```python
from build123d import *

# Parameters (mm, degrees)
F0_R     = 6.35
F1_DEPTH = 25.4
F2_SIZE  = 6.35
F3_W     = 63.5
F3_H     = 19.05
F4_DEPTH = 95.25
F5_R     = 6.35
F7_DEPTH = 50.801


with BuildPart() as f1:
    # F0 (on Top) → F1 (new body)
    with BuildSketch(Plane.XY):
        with BuildLine():
            ThreePointArc((0, 15.875), (4.6496798487, 4.6496798487), (15.875, 0))
            Line((15.875, 0), (60.325, 0))
            ThreePointArc((60.325, 0), (71.5503201513, 4.6496798487), (76.2, 15.875))
            Line((76.2, 15.875), (76.2, 85.725))
            ThreePointArc((76.2, 85.725), (71.5503201513, 96.9503201513), (60.325, 101.6))
            Line((60.325, 101.6), (15.875, 101.6))
            ThreePointArc((15.875, 101.6), (4.6496798487, 96.9503201513), (0, 85.725))
            Line((0, 85.725), (0, 15.875))
        make_face()
        with Locations((15.875, 15.875)):
            Circle(F0_R, mode=Mode.SUBTRACT)
        with Locations((60.325, 15.875)):
            Circle(F0_R, mode=Mode.SUBTRACT)
        with Locations((15.875, 85.725)):
            Circle(F0_R, mode=Mode.SUBTRACT)
        with Locations((60.325, 85.725)):
            Circle(F0_R, mode=Mode.SUBTRACT)
    extrude(amount=F1_DEPTH)

    # F2
    f2_edges = [f1.edges().sort_by_distance(p)[0] for p in [
        (38.1, 0, 25.4),
        (0, 50.8, 25.4),
        (4.64968, 4.64968, 25.4),
        (71.55032, 4.64968, 25.4),
        (76.2, 50.8, 25.4),
        (71.55032, 96.95032, 25.4),
        (38.1, 101.6, 25.4),
        (4.64968, 96.95032, 25.4),
    ]]
    chamfer(f2_edges, length=F2_SIZE)

    # F3 (on face) → F4 (join)
    with BuildSketch(Plane.XY.offset(25.4)):
        with Locations((38.1, 60.325)):
            Rectangle(F3_W, F3_H)
    extrude(amount=F4_DEPTH)

    # F5
    f5_edges = [f1.edges().sort_by_distance(p)[0] for p in [
        (38.1, 50.8, 25.4),
        (38.1, 69.85, 25.4),
    ]]
    fillet(f5_edges, radius=F5_R)

    # F6 (on face) → F7 (cut, through all)
    with BuildSketch(Plane.XZ.offset(-50.8)):
        with BuildLine():
            Line((6.35, 120.65), (6.35, 61.0775296334))
            ThreePointArc((6.35, 61.0775296334), (9.7019366858, 75.2765612905), (19.05, 86.4775296334))
            Line((19.05, 86.4775296334), (19.05, 120.65))
            Line((19.05, 120.65), (6.35, 120.65))
        make_face()
        with BuildLine():
            ThreePointArc((57.15, 61.0775296334), (38.1, 80.1275296334), (19.05, 61.0775296334))
            Line((19.05, 61.0775296334), (38.1, 61.0775296334))
            Line((38.1, 61.0775296334), (38.1, 42.0275296334))
            ThreePointArc((38.1, 42.0275296334), (51.5703841816, 47.6071454518), (57.15, 61.0775296334))
        make_face()
        with BuildLine():
            Line((19.05, 86.4775296334), (19.05, 61.0775296334))
            ThreePointArc((19.05, 61.0775296334), (38.1, 80.1275296334), (57.15, 61.0775296334))
            Line((57.15, 61.0775296334), (57.15, 86.4775296334))
            ThreePointArc((57.15, 86.4775296334), (38.1, 92.8275296334), (19.05, 86.4775296334))
        make_face()
        with BuildLine():
            Line((38.1, 61.0775296334), (19.05, 61.0775296334))
            ThreePointArc((19.05, 61.0775296334), (24.6296158184, 47.6071454518), (38.1, 42.0275296334))
            Line((38.1, 42.0275296334), (38.1, 61.0775296334))
        make_face()
        with BuildLine():
            Line((19.05, 120.65), (19.05, 86.4775296334))
            ThreePointArc((19.05, 86.4775296334), (38.1, 92.8275296334), (57.15, 86.4775296334))
            Line((57.15, 86.4775296334), (57.15, 120.65))
            Line((57.15, 120.65), (19.05, 120.65))
        make_face()
        with BuildLine():
            ThreePointArc((57.15, 86.4775296334), (66.4980633142, 75.2765612905), (69.85, 61.0775296334))
            Line((69.85, 61.0775296334), (69.85, 120.65))
            Line((69.85, 120.65), (57.15, 120.65))
            Line((57.15, 120.65), (57.15, 86.4775296334))
        make_face()
    extrude(amount=-F7_DEPTH, mode=Mode.SUBTRACT)


solid = f1.part
```
Source: CAD feature listing. Evaluate the final solid. Frame: model axes, mm. A direction names the side the tool comes from. Coordinates: 2 decimals unless noted, no trailing zeros. Order: outer loops, then holes, each group sorted by start corner. A loop starts at its lowest first (then second) coordinate and runs counter-clockwise, first axis right, second up. Notation, with made-up numbers: (-16, -8) - (7, -8) arc R22 cw to (7, 5) - close; hole circle Ø1 at (-22, 28.5). An arc over 180 degrees is marked (long way). One line per item, written item: value.
1) Cut plane D-D on x = 23.5. Output: boundary loops of the cut face in (y, z).
Computed values:
outline: (0, 0) - (101.6, 0) - (101.6, 19.05) - (95.25, 25.4) - (76.2, 25.4) arc R6.35 cw to (69.85, 31.75) - (69.85, 48.84) - (50.8, 48.84) - (50.8, 31.75) arc R6.35 cw to (44.45, 25.4) - (6.35, 25.4) - (0, 19.05) - close
2) Mould query, pull axis X, two halves, no side actions, for faces 1 (the face through (76.2, 50, 9)), 2 (the face through (38.41, 98.38, 22.27)), 3 (the face through (9.61, 60.19, 75.09)), 4 (the face through (66.19, 13.44, 12.52)). Classes: released by +X, released by -X, zero draft, split by the parting line, or undercut.
Computed values:
face 1: released by +X
face 2: zero draft
face 3: released by -X
face 4: undercut
3) Ray query, line 1 (X direction, y = 21, z = 22); line 2 (Z direction, x = 73, y = 55.5); line 3 (X direction, y = 62.5, z = 48). Return the intervals inside material, ascending. Write a range as [from, to].
Computed values:
line 1: x = [2.95, 12.13], [19.62, 56.58], [64.07, 73.25]
line 2: z = [0, 22.25]
line 3: x = [6.35, 24.25], [51.95, 69.85]
4) Cut plane A-A on z = 6.5. Output: boundary loops of the cut face in (x, y) (3 decimals), plus the area to 3 significant figures.
Computed values:
outline: (0, 15.875) arc R15.875 ccw to (15.875, 0) - (60.325, 0) arc R15.875 ccw to (76.2, 15.875) - (76.2, 85.725) arc R15.875 ccw to (60.325, 101.6) - (15.875, 101.6) arc R15.875 ccw to (0, 85.725) - close; hole circle Ø12.7 at (15.875, 15.875); hole circle Ø12.7 at (15.875, 85.725); hole circle Ø12.7 at (60.325, 15.875); hole circle Ø12.7 at (60.325, 85.725)
area: 7,020 mm^2
5) Cut plane C-C on y = 55.5. Output: boundary loops of the cut face in (x, z), plus the area to 3 significant figures.
Computed values:
outline: (0, 0) - (76.2, 0) - (76.2, 19.05) - (69.85, 25.4) - (69.85, 61.08) arc R31.75 ccw to (57.15, 86.48) - (57.15, 61.08) arc R19.05 cw to (19.05, 61.08) - (19.05, 86.48) arc R31.75 ccw to (6.35, 61.08) - (6.35, 25.4) - (0, 19.05) - close
area: 4,040 mm^2
6) Contact query for flat-ended pins moving along their axis: pin 1 (16.5 mm diameter, centred on x = 40.5, z = 46.5, fed in from +Y); pin 2 (21 mm diameter, centred on x = 34.5, y = 88, fed in from +Z); pin 3 (7.5 mm diameter, centred on x = 60.325, y = 85.725, fed in from +Z); pin 4 (12 mm diameter, centred on x = 49.5, y = 72, fed in from +Z). Output: stop coordinate, or through.
Computed values:
pin 1: stops at y = 69.85
pin 2: stops at z = 25.4
pin 3: passes through
pin 4: stops at z = 52.48
7) Reachability of faces 5 (the face through (38, 50.8, 40)), 6 (the face through (68.867, 94.082, 22.975)), 7 (the face through (69.85, 60, 43)) from +Z, -Z, +X, -X, +Y, -Y: full face, straight path, thin tool, end or side. Return the list, or none.
Computed values:
face 5: +Z, +X, -X, -Y
face 6: +Z, +X, +Y
face 7: +Z, +X, +Y, -Y
8) Cut plane B-B on z = 74. Output: boundary loops of the cut face in (x, y), plus the area to 3 significant figures.
Computed values:
outline: (9.1, 50.8) - (19.05, 50.8) - (19.05, 69.85) - (9.1, 69.85) - close; (57.15, 50.8) - (67.1, 50.8) - (67.1, 69.85) - (57.15, 69.85) - close
area: 379 mm^2
